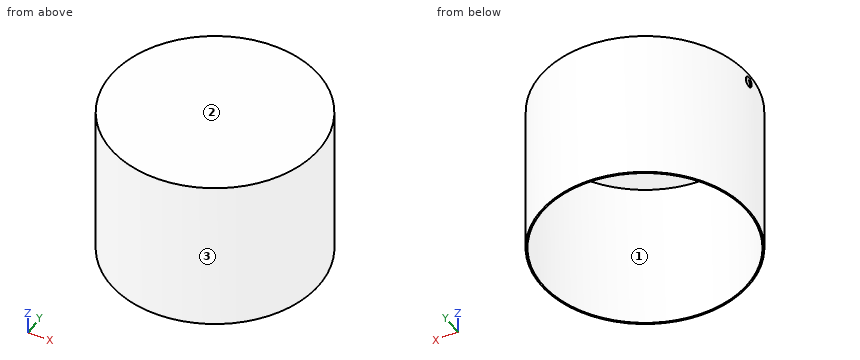
from build123d import *

# Parameters (mm, degrees)
SKETCH1_R           = 103.1875
BOSS_EXTRUDE1_DEPTH = 152.4
SKETCH2_R           = 101.6
CUT_EXTRUDE1_DEPTH  = 149.225
SKETCH3_R           = 5.08
CUT_EXTRUDE2_DEPTH  = 212.000190314


with BuildPart() as part:
    # Sketch1 → Boss-Extrude1 (new body)
    with BuildSketch(Plane.XY):
        with Locations(Location((0, 0, 0), (0, 0, 180))):
            Circle(SKETCH1_R)
    extrude(amount=BOSS_EXTRUDE1_DEPTH)

    # Sketch2 → Cut-Extrude1 (cut)
    with BuildSketch(Plane(origin=(0, 0, 0), x_dir=(-1, 0, 0), z_dir=(0, 0, -1))):
        Circle(SKETCH2_R)
    extrude(amount=-CUT_EXTRUDE1_DEPTH, mode=Mode.SUBTRACT)

    # Sketch3 → Cut-Extrude2 (cut, through all)
    with BuildSketch(Plane(origin=(0, 0, 0), x_dir=(0, 0, -1), z_dir=(1, 0, 0))):
        with Locations((-144.145, 0)):
            Circle(SKETCH3_R)
    extrude(amount=-CUT_EXTRUDE2_DEPTH, mode=Mode.SUBTRACT)


solid = part.part
For this review, take the finished solid that the model builds, in its own axes (mm). Face numbers are marked on the shaded views. Round coordinates to 2 decimals unless told otherwise and drop trailing zeros. Loops run counter-clockwise (first coordinate to the right, second up) from the corner with the lowest first, then second, coordinate; pieces in that order, holes last. Notation, with made-up numbers: (42.25, 79.25) - (79.25, 79.25) arc R21 cw to (79.25, 112.25) - close; hole circle Ø2 at (59.25, 46). An arc over 180 degrees is marked (long way). Answer as CSV lines item,"result".
(1) Insertion check: P1, Ø6, axis at x = -52, z = 88, coming from the -Y side; P2, Ø6, axis at x = -13.5, z = 111, coming from the +Y side; P3, Ø3, axis at x = 17, z = 94, coming from the -Y side. Each pin has a flat end and moves straight along its axis. Give the tip position at first contact, or say it passes through.
Checked values:
P1,"stops at y = -90.81"
P2,"stops at y = 102.65"
P3,"stops at y = -102.02"
(2) Mouldability with a two-part tool opening along Y and no side actions: class the marked faces 1, 2 and 3 as +Y half, -Y half, draft (parallel to the pull), parting line (faces both ways), or undercut.
Checked values:
face 1,"undercut"
face 2,"draft"
face 3,"parting line"
(3) Consider section C-C on z = 59. Give the boundary of the cut face in (x, y) (1 decimal).
Checked values:
outline,"circle Ø206.4 at (0, 0); hole circle Ø203.2 at (0, 0)"
(4) Wall thickness on line 1 (Z direction, x = -102.65, y = 0) (3 decimals); line 2 (Y direction, x = 0, z = 60.5); line 3 (Z direction, x = -88, y = -15.5) (3 decimals): over which ranges is each line inside the solid? List them lowest first.
Checked values:
line 1,"z = 0 to 139.065, 149.225 to 152.4"
line 2,"y = -103.19 to -101.6, 101.6 to 103.19"
line 3,"z = 149.225 to 152.4"
(5) Consider section B-B on y = 13. Give the boundary of the cut face in (x, z) (3 decimals).
Checked values:
outline,"(-102.365, 0) - (-100.765, 0) - (-100.765, 149.225) - (100.765, 149.225) - (100.765, 0) - (102.365, 0) - (102.365, 152.4) - (-102.365, 152.4) - close"
(6) Consider section A-A on x = 0. Give the boundary of the cut face in (y, z) (1 decimal).
Checked values:
outline,"(-103.2, 0) - (-101.6, 0) - (-101.6, 149.2) - (101.6, 149.2) - (101.6, 0) - (103.2, 0) - (103.2, 152.4) - (-103.2, 152.4) - close"
